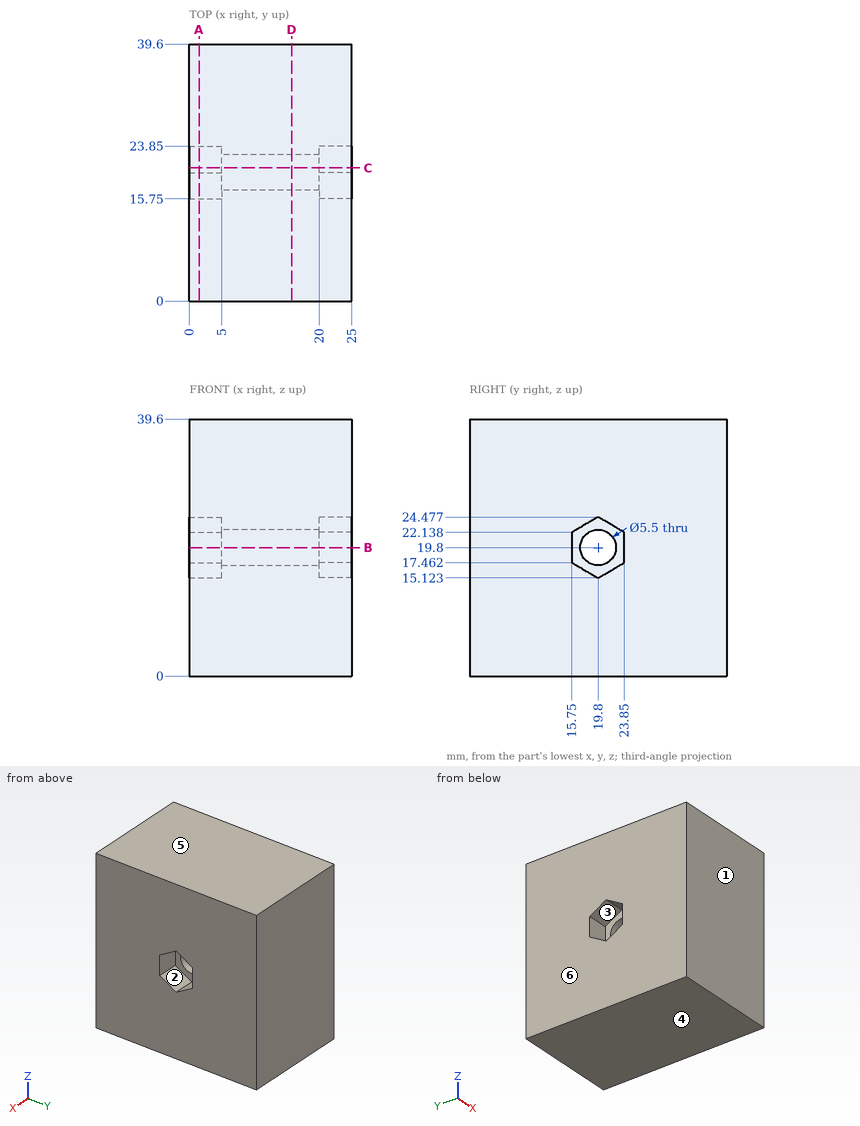
Verification items for this drawing (mm, ordinates from the low corner). A direction names the side the tool comes from. Coordinates: 2 decimals unless noted, no trailing zeros. Write each loop counter-clockwise with the first axis right and the second up, starting at its lowest first coordinate (ties: lowest second). Pieces come first, ordered by that corner, then holes. Notation, with made-up numbers: M 27,80 L 42,80 A17 cw 42,85 Z; hole C 72,12.5 d7. An arc over 180 degrees is marked long. Answer as a JSON object with one key per item and string values. Group by question number.
(1) Cross-section at D-D, the plane x = 15.75. Record the cut outline in (y, z).
(2) Material ranges on line 1 (Z direction, x = 9.5, y = 19.8); line 2 (Y direction, x = 16.5, z = 18), recorded low to high.
(3) Release check for a two-part mould opening along Z. For the marked faces 3, 4, 5 and 6 record: +Z half, -Z half, draft (parallel to the pull), parting line (faces both ways), or undercut.
(4) Cross-section at B-B, the plane z = 19.8. Record the cut outline in (x, y).
(5) Gauge pin test, flat ends, axial feed: pin 1 (3.5 mm diameter, centred on y = 19.8, z = 19.8, fed in from +X); pin 2 (2.5 mm diameter, centred on y = 21, z = 17.5, fed in from -X); pin 3 (8 mm diameter, centred on x = 11, z = 7, fed in from -Y). Record the tip position at first contact, or that the pin passes through.
(6) Cross-section at A-A, the plane x = 1.5. Record the cut outline in (y, z).
(7) Cross-section at C-C, the plane y = 20.5. Record the cut outline in (x, z).
(8) Tool access check on the marked faces 1 and 2. Record the directions out of +Z, -Z, +X, -X, +Y, -Y that give a thin tool (end or side, any length) a straight path to the whole face; none if there is none.
Reply:
{
 "1": {"outline": "M 0,0 L 39.6,0 L 39.6,39.6 L 0,39.6 Z; hole C 19.8,19.8 d5.5"},
 "2": {"line 1": "0 to 17.05, 22.55 to 39.6", "line 2": "0 to 17.72, 21.88 to 39.6"},
 "3": {"face 3": "undercut", "face 4": "-Z half", "face 5": "+Z half", "face 6": "draft"},
 "4": {"outline": "M 0,0 L 25,0 L 25,15.75 L 20,15.75 L 20,17.05 L 5,17.05 L 5,15.75 L 0,15.75 Z; M 0,23.85 L 5,23.85 L 5,22.55 L 20,22.55 L 20,23.85 L 25,23.85 L 25,39.6 L 0,39.6 Z"},
 "5": {"pin 1": "through", "pin 2": "x = 5", "pin 3": "y = 0"},
 "6": {"outline": "M 0,0 L 39.6,0 L 39.6,39.6 L 0,39.6 Z; hole M 15.75,17.46 L 19.8,15.12 L 23.85,17.46 L 23.85,22.14 L 19.8,24.48 L 15.75,22.14 Z"},
 "7": {"outline": "M 0,0 L 25,0 L 25,15.53 L 20,15.53 L 20,17.14 L 5,17.14 L 5,15.53 L 0,15.53 Z; M 0,24.07 L 5,24.07 L 5,22.46 L 20,22.46 L 20,24.07 L 25,24.07 L 25,39.6 L 0,39.6 Z"},
 "8": {"face 1": "+Z, -Z, +X, -X, -Y", "face 2": "+X"}
}
